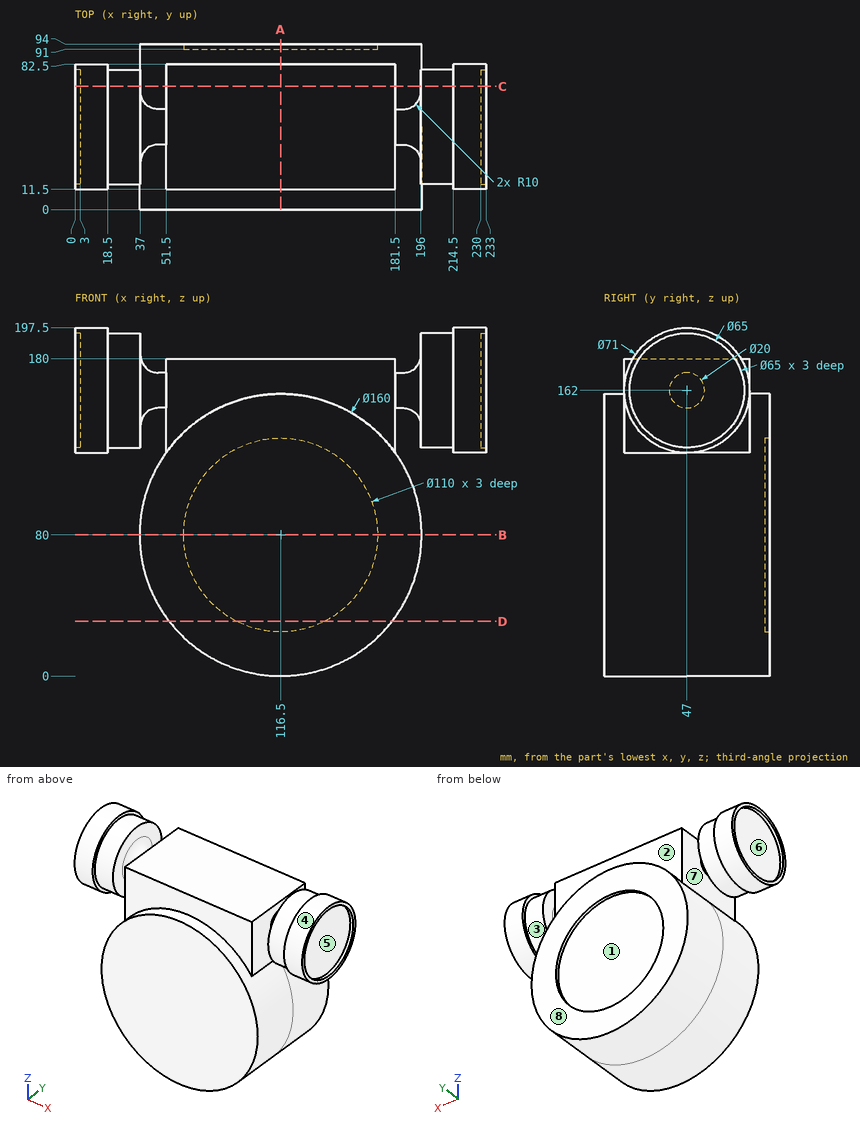
Part print with two shaded views. Sizes in mm from the minimum x, y, z corner. A direction names the side the tool comes from. Give positions to 0.01 mm unless a question says otherwise; leave off trailing zeros. Write each loop counter-clockwise with the first axis right and the second up, starting at its lowest first coordinate (ties: lowest second). Pieces come first, ordered by that corner, then holes.
1) Two-plate mould, pull along Y, no slides. Class the marked faces 5, 6, 7 and 8: released by +Y, released by -Y, zero draft, split by the parting line, or undercut.
Resolved:
face 5: undercut
face 6: undercut
face 7: zero draft
face 8: released by +Y
2) Pin check, flat tips, straight feed: pin 1 (4 mm diameter, centred on y = 44, z = 43.5, fed in from -X); pin 2 (6 mm diameter, centred on x = 147, y = 32.5, fed in from -Z); pin 3 (10 mm diameter, centred on x = 195.5, y = 41.5, fed in from +Z). Stop position of each tip, or through.
Resolved:
pin 1: stops at x = 44.32
pin 2: stops at z = 4.88
pin 3: stops at z = 194.5
3) Which spindle directions (+Z, -Z, +X, -X, +Y, -Y) get a long thin tool onto all of the face, cutting with end or side? Do the marked faces 1, 2, 3 and 4. Say none if no direction does.
Resolved:
face 1: +Y
face 2: +Z, +Y
face 3: none
face 4: +X
4) Cut at C-C on y = 70. Write the cut outline in (x, z).
Resolved:
outline: (0, 134.96) - (18.5, 134.96) - (18.5, 139.04) - (37, 139.04) - (37, 184.96) - (18.5, 184.96) - (18.5, 189.04) - (0, 189.04) - (0, 184.96) - (3, 184.96) - (3, 139.04) - (0, 139.04) - close; (51.5, 126.64) arc R80 ccw (long way) to (181.5, 126.64) - (181.5, 180) - (51.5, 180) - close; (196, 139.04) - (214.5, 139.04) - (214.5, 134.96) - (233, 134.96) - (233, 139.04) - (230, 139.04) - (230, 184.96) - (233, 184.96) - (233, 189.04) - (214.5, 189.04) - (214.5, 184.96) - (196, 184.96) - close
5) Cut at D-D on z = 31. Write the cut outline in (x, y).
Resolved:
outline: (53.26, 0) - (179.74, 0) - (179.74, 94) - (141.48, 94) - (141.48, 91) - (91.52, 91) - (91.52, 94) - (53.26, 94) - close
6) Cut at B-B on z = 80. Write the cut outline in (x, y), then the cut area to 3 significant figures.
Resolved:
outline: (36.5, 0) - (196.5, 0) - (196.5, 94) - (171.5, 94) - (171.5, 91) - (61.5, 91) - (61.5, 94) - (36.5, 94) - close
area: 14,700 mm2
7) Cut at A-A on x = 116.5. Write the cut outline in (y, z).
Resolved:
outline: (0, 0) - (94, 0) - (94, 25) - (91, 25) - (91, 135) - (94, 135) - (94, 160) - (82.5, 160) - (82.5, 180) - (11.5, 180) - (11.5, 160) - (0, 160) - close
8) Probe L1, parallel to X at y = 64, z = 179; L2, parallel to X at y = 43, z = 128; L3, parallel to Y at x = 231.15, z = 162. List the from-to ranges inside material, lowest first.
Resolved:
L1: x = 3 to 37, 51.5 to 181.5, 196 to 230
L2: x = 0 to 18.5, 51.5 to 181.5, 214.5 to 233
L3: y = 11.5 to 14.5, 79.5 to 82.5
